from build123d import *

# Parameters (mm, degrees)
ESBO_O1_R                = 1.7
ESBO_O1_W                = 58
ESBO_O1_H                = 35
RESSALTO_EXTRUS_O1_DEPTH = 3
ESBO_O2_R                = 2.1
RESSALTO_EXTRUS_O2_DEPTH = 3
ESBO_O3_W                = 3
ESBO_O3_H                = 35
EXTRUS_O_FINA1_DEPTH     = 3


with BuildPart() as part:
    # Esboço1 → Ressalto-extrusão1 (new body)
    with BuildSketch(Plane.XY):
        with BuildLine():
            Line((92.5, 23.5), (-92.5, 23.5))
            ThreePointArc((-92.5, 23.5), (-95.5, 20.5), (-92.5, 17.5))
            Line((-92.5, 17.5), (-49, 17.5))
            Line((-49, 17.5), (-49, -17.5))
            Line((-49, -17.5), (-92.5, -17.5))
            ThreePointArc((-92.5, -17.5), (-95.5, -20.5), (-92.5, -23.5))
            Line((-92.5, -23.5), (92.5, -23.5))
            ThreePointArc((92.5, -23.5), (95.5, -20.5), (92.5, -17.5))
            Line((92.5, -17.5), (21, -17.5))
            Line((21, -17.5), (21, 17.5))
            Line((21, 17.5), (92.5, 17.5))
            ThreePointArc((92.5, 17.5), (95.5, 20.5), (92.5, 23.5))
        make_face()
        with Locations((-92.5, 20.5)):
            Circle(ESBO_O1_R, mode=Mode.SUBTRACT)
        with Locations((92.5, 20.5)):
            Circle(ESBO_O1_R, mode=Mode.SUBTRACT)
        with Locations((18, 20.5)):
            Circle(ESBO_O1_R, mode=Mode.SUBTRACT)
        with Locations((-46, 20.5)):
            Circle(ESBO_O1_R, mode=Mode.SUBTRACT)
        with Locations((-46, -20.5)):
            Circle(ESBO_O1_R, mode=Mode.SUBTRACT)
        with Locations((18, -20.5)):
            Circle(ESBO_O1_R, mode=Mode.SUBTRACT)
        with Locations((92.5, -20.5)):
            Circle(ESBO_O1_R, mode=Mode.SUBTRACT)
        with Locations((-92.5, -20.5)):
            Circle(ESBO_O1_R, mode=Mode.SUBTRACT)
        with Locations((-14, 0)):
            Rectangle(ESBO_O1_W, ESBO_O1_H, mode=Mode.SUBTRACT)
    extrude(amount=RESSALTO_EXTRUS_O1_DEPTH)

    # Esboço2 → Ressalto-extrusão2 (add)
    with BuildSketch(Plane.XY.offset(3)):
        with BuildLine():
            Line((21, 23.5), (15, 23.5))
            ThreePointArc((15, 23.5), (18, 16.257359313), (21, 23.5))
        make_face()
        with Locations((18, 20.5)):
            Circle(ESBO_O2_R, mode=Mode.SUBTRACT)
        with BuildLine():
            Line((-49, -23.5), (-43, -23.5))
            ThreePointArc((-43, -23.5), (-46, -16.257359313), (-49, -23.5))
        make_face()
        with Locations((-46, -20.5)):
            Circle(ESBO_O2_R, mode=Mode.SUBTRACT)
        with BuildLine():
            Line((-43, 23.5), (-49, 23.5))
            ThreePointArc((-49, 23.5), (-46, 16.257359313), (-43, 23.5))
        make_face()
        with Locations((-46, 20.5)):
            Circle(ESBO_O2_R, mode=Mode.SUBTRACT)
        with BuildLine():
            Line((15, -23.5), (21, -23.5))
            ThreePointArc((21, -23.5), (18, -16.257359313), (15, -23.5))
        make_face()
        with Locations((18, -20.5)):
            Circle(ESBO_O2_R, mode=Mode.SUBTRACT)
    extrude(amount=RESSALTO_EXTRUS_O2_DEPTH)

    # Esboço3 → Extrusão-Fina1 (add, through all)
    with BuildSketch(Plane.XY.offset(3)):
        with Locations((-85, 0)):
            Rectangle(ESBO_O3_W, ESBO_O3_H)
        with Locations((85, 0)):
            Rectangle(ESBO_O3_W, ESBO_O3_H)
    extrude(amount=-EXTRUS_O_FINA1_DEPTH)


solid = part.part
CAD build for the part. Positions are in the model's coordinates, mm. A direction names the side the tool comes from. Give positions to 0.01 mm unless a question says otherwise; leave off trailing zeros. Write each loop counter-clockwise with the first axis right and the second up, starting at its lowest first coordinate (ties: lowest second). Pieces come first, ordered by that corner, then holes. Notation, with made-up numbers: (35, -12) -> (69, -12) arc R25 cw to (69, 8) -> close; hole circle Ø8 at (25.5, -12). An arc over 180 degrees is marked (long way). Return JSON: item names as keys, results as strings.
Item 1: Drill centre lines: probe 1 along Y at (x, z) = (-92.5, 0.7); probe 2 along Y at (x, z) = (18, 4.05); probe 3 along X at (y, z) = (5.5, 1.1). Where is each one in solid material? Low to high.
Answer below:
{"probe 1": "y = -23.5 to -22.2, -18.8 to -17.5, 17.5 to 18.8, 22.2 to 23.5", "probe 2": "y = -23.5 to -22.6, -18.4 to -16.26, 16.26 to 18.4, 22.6 to 23.5", "probe 3": "x = -86.5 to -83.5, -49 to -43, 15 to 21, 83.5 to 86.5"}
Item 2: Tool access for faces 1 (the flat face through (-89, -17.5, 1)), 2 (the flat face through (89, 17.5, 1)), 3 (the cylindrical face through (17.86, 16.26, 4.48)), 4 (the flat face through (1, 23.5, 2)), 5 (the flat face through (-49, 0, 1)): list every direction of +Z, -Z, +X, -X, +Y, -Y with a clear straight run to the whole face (end or side of a thin tool).
Answer below:
{"face 1": "+Z, -Z, -X", "face 2": "+Z, -Z, +X", "face 3": "+Z", "face 4": "+Z, -Z, +X, -X, +Y", "face 5": "+Z, -Z"}
Item 3: Band-saw the part on C-C (y = -13.5). List the corners of the cut face in (x, z).
Answer below:
{"outline": "(-86.5, 0) -> (-83.5, 0) -> (-83.5, 3) -> (-86.5, 3) -> close; (-49, 0) -> (-43, 0) -> (-43, 3) -> (-49, 3) -> close; (15, 0) -> (21, 0) -> (21, 3) -> (15, 3) -> close; (83.5, 0) -> (86.5, 0) -> (86.5, 3) -> (83.5, 3) -> close"}
Item 4: Drop flat-ended pins along their axis: pin 1 (4 mm diameter, centred on x = -92.5, y = 20.5, fed in from +Z); pin 2 (1.5 mm diameter, centred on y = 4.5, z = 1, fed in from -X); pin 3 (3 mm diameter, centred on x = -46, y = -20.5, fed in from +Z); pin 4 (1.5 mm diameter, centred on y = 7.5, z = 1, fed in from +X). Give the stop position or say it passes through.
Answer below:
{"pin 1": "stops at z = 3", "pin 2": "stops at x = -86.5", "pin 3": "passes through", "pin 4": "stops at x = 86.5"}
Item 5: Band-saw the part on B-B (z = 0.9). Give the number of separate pieces and of enclosed holes in the cut face, then the cut area to 3 significant figures.
Answer below:
{"separate pieces": "1", "enclosed holes": "11", "area": "2,830 mm2"}
Item 6: Band-saw the part on A-A (x = -46). List the corners of the cut face in (y, z).
Answer below:
{"outline": "(-23.5, 0) -> (-22.2, 0) -> (-22.2, 3) -> (-22.6, 3) -> (-22.6, 6) -> (-23.5, 6) -> close; (-18.8, 0) -> (18.8, 0) -> (18.8, 3) -> (18.4, 3) -> (18.4, 6) -> (16.26, 6) -> (16.26, 3) -> (-16.26, 3) -> (-16.26, 6) -> (-18.4, 6) -> (-18.4, 3) -> (-18.8, 3) -> close; (22.2, 0) -> (23.5, 0) -> (23.5, 6) -> (22.6, 6) -> (22.6, 3) -> (22.2, 3) -> close"}
